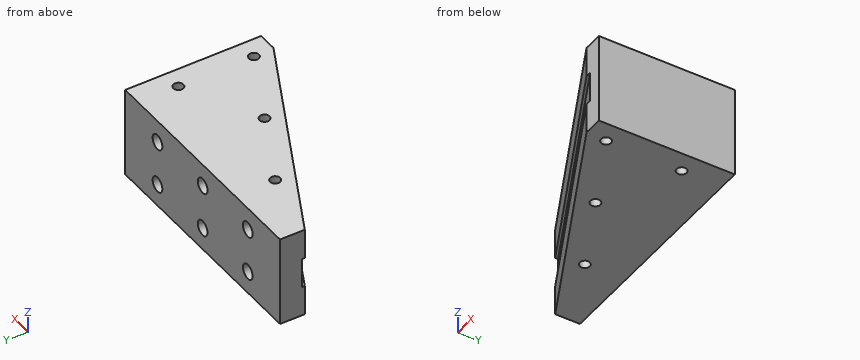
Autodesk Inventor part; units mm, degrees
ref_plane "Work Plane1" through (21.5154, -24.3167, -9) normal (-0.4472, -0.8944, 0) x (0.8944, -0.4472, 0)
ref_plane "YZ Plane" through (0, 0, 0) normal (1, 0, 0) x (0, 1, 0)
ref_plane "XZ Plane" through (0, 0, 0) normal (0, 1, 0) x (-1, 0, 0)
sketch "Sketch2" plane through (0, 0, 0) normal (0, 0, 1) x (1, 0, 0)
  line L0 (20, -8) -> (-10, -8) construction
  line L1 (-10, -8) -> (-10, -23) construction
  line L2 (-10, -23) -> (20, -23) construction
  line L3 (20, -23) -> (20, -8) construction
  line L4 (20, -8) -> (-10, -23) construction
  line L5 (-10, -8) -> (20, -23) construction
  point P0 (5, -15.5)
  point P1 (5, -15.5)
  point P2 (0, 0)
  dimension "d2" = 30
  dimension "d3" = 15
  dimension "d4" = 5
  dimension "d5" = 8
sketch "Sketch3" plane through (0, 0, 0) normal (0, 0, 1) x (1, 0, 0)
  line L0 (24, 0) -> (24, -27)
  line L1 (24, -27) -> (20.1738, -27)
  line L2 (20.1738, -27) -> (-24, -4.9131)
  line L3 (-24, -4.9131) -> (-24, 0)
  line L4 (-24, 0) -> (24, 0)
  line L5 (20, -23) -> (-10, -8) construction
  point P0 (0, 0)
  point P1 (5, -15.5)
  point P2 (20, -8)
  dimension "d6" = 4
  dimension "d8" = 3.5
  dimension "d9" = 4
extrude "Extrusion1" add sketch "Sketch3" along normal mid plane 18
sketch "Sketch4" plane through (0, 0, 9) normal (0, 0, 1) x (1, 0, 0)
  point P0 (0, 0)
  point P1 (20, -23)
  point P2 (5, -15.5)
  point P3 (-10, -8)
  point P4 (20, -8)
hole "Hole1" at (20, -23, 9) at (5, -15.5, 9) at (-10, -8, 9) at (20, -8, 9) direction (0, 0, -1) diameter 2 end through all
ref_plane "Work Plane1" through (21.5154, -24.3167, -9) normal (-0.4472, -0.8944, 0) x (0.8944, -0.4472, 0)
sketch "Sketch9" plane through (20.1738, -27, -9) normal (-0.4472, -0.8944, 0) x (0.8944, -0.4472, 0)
  line L0 (19.8813, 12) -> (-80.1187, 12)
  line L1 (-80.1187, 12) -> (-80.1187, 6)
  line L2 (-80.1187, 6) -> (19.8813, 6)
  line L3 (19.8813, 6) -> (19.8813, 12)
  line L4 (19.8813, 12) -> (-80.1187, 6) construction
  line L5 (-80.1187, 12) -> (19.8813, 6) construction
  point P0 (-30.1187, 9)
  dimension "d54" = 6
  dimension "d55" = 100
extrude "Extrusion2" cut sketch "Sketch9" against normal blind 0.5
sketch "Sketch10" plane through (-24, 0, 9) normal (0, 1, 0) x (1, 0, 0)
  line L0 (24, 9) -> (42.9051, 9) construction
  point P0 (24, 13.5)
  point P1 (24, 4.5)
  point P2 (10, 13.5)
  point P3 (10, 4.5)
  point P4 (38, 4.5)
  point P5 (38, 13.5)
  dimension "d58" = 9
  dimension "d59" = 14
  dimension "d60" = 14
hole "Hole6" at (0, 0, -4.5) at (0, 0, 4.5) at (-14, 0, -4.5) at (-14, 0, 4.5) at (14, 0, 4.5) at (14, 0, -4.5) direction (0, -1, 0) diameter 3 depth 8 tip angle 118
properties part number "wrist adapter"
For this review, take the finished solid that the model builds, in its own axes (mm). Round coordinates to 2 decimals unless told otherwise and drop trailing zeros. Loops run counter-clockwise (first coordinate to the right, second up) from the corner with the lowest first, then second, coordinate; pieces in that order, holes last. Notation, with made-up numbers: (8, -1.5) - (32, -1.5) arc R13 cw to (32, 13.5) - close; hole circle Ø1 at (-12, 52). An arc over 180 degrees is marked (long way). Put each result on its own line as item: value. Start each with the question number.
1. Consider section C-C on y = -15.5. State the section outline as (x, z) points, plus the area to 3 significant figures.
2. Consider section D-D on x = -10. State the section outline as (y, z) points.
3. For probe 1 along X at (y, z) = (-2, 4.5); probe 2 along Z at (x, y) = (14, -3.5); probe 3 along Y at (x, z) = (20, -3.75), list the stretches that pass through material, from the lowest coordinate up. Write a range as [from, to].
4. Consider section A-A on z = 7.25. State the section outline as (x, y) points, plus the area to 3 significant figures.
5. Insertion check: P1, Ø4, axis at x = -14, z = 4.5, coming from the -Y side; P2, Ø3, axis at x = 5.5, z = 5, coming from the -Y side; P3, Ø2.5, axis at x = -14, z = -4.5, coming from the -Y side; P4, Ø3, axis at x = -10, y = -8, coming from the +Z side. Each pin has a flat end and moves straight along its axis. Give the tip position at first contact, or say it passes through.
6. Consider section B-B on y = -2.5. State the section outline as (x, z) points.
Result sheet:
1. outline: (-2.83, -9) - (4, -9) - (4, 9) - (-2.83, 9) - (-2.83, 3) - (-1.7, 3) - (-1.7, -3) - (-2.83, -3) - close; (6, -9) - (24, -9) - (24, 9) - (6, 9) - close
1. area: 440 mm^2
2. outline: (-11.91, -9) - (-9, -9) - (-9, 9) - (-11.91, 9) - (-11.91, 3) - (-11.35, 3) - (-11.35, -3) - (-11.91, -3) - close; (-7, -9) - (0, -9) - (0, 9) - (-7, 9) - close
3. probe 1: [-24, -15.5], [-12.5, -1.5], [1.5, 12.5], [15.5, 24]
3. probe 2: [-9, -6], [-3, 3], [6, 9]
3. probe 3: [-26.91, -24], [-22, -9], [-7, 0]
4. outline: (-24, -4.91) - (20.17, -27) - (24, -27) - (24, 0) - (-24, 0) - close; hole circle Ø2 at (-10, -8); hole circle Ø2 at (5, -15.5); hole circle Ø2 at (20, -23); hole circle Ø2 at (20, -8)
4. area: 796 mm^2
5. P1: y = -10.91
5. P2: y = -20.41
5. P3: y = -10.54
5. P4: z = 9
6. outline: (-24, -9) - (24, -9) - (24, 9) - (-24, 9) - close; hole circle Ø3 at (-14, -4.5); hole circle Ø3 at (-14, 4.5); hole circle Ø3 at (0, -4.5); hole circle Ø3 at (0, 4.5); hole circle Ø3 at (14, -4.5); hole circle Ø3 at (14, 4.5)
